```python
from build123d import *

# Parameters (mm, degrees)
BOSS_EXTRUDE1_DEPTH       = 10.287
SKETCH2_R                 = 3.556
CUT_EXTRUDE1_DEPTH        = 0.635
SKETCH3_W                 = 3.048
SKETCH3_H                 = 6.858
CUT_EXTRUDE2_DEPTH        = 0.635
SKETCH4_W                 = 6.731
SKETCH4_H                 = 1.016
CUT_EXTRUDE3_DEPTH        = 1.016
SKETCH5_W                 = 2.54
SKETCH5_H                 = 6.35
CUT_EXTRUDE4_DEPTH        = 0.635
FILLET1_R                 = 6.35
FILLET2_R                 = 2.54
CUT_EXTRUDE5_DEPTH        = 66.856694641
SKETCH9_W                 = 2.54
SKETCH9_H                 = 6.35
SKETCH9_R                 = 3.556
BOSS_EXTRUDE2_DEPTH       = 0.635
SKETCH10_W                = 6.731
SKETCH10_H                = 1.016
BOSS_EXTRUDE3_DEPTH       = 1.016
SKETCH12_W                = 3.048
SKETCH12_H                = 6.858
BOSS_EXTRUDE4_DEPTH       = 1.27
FILLET5_R                 = 0.508
FILLET5_OF_MIRROR4_R      = 0.508
F_1_0_16_DIAMETER_HOLE1_D = 4.064
SKETCH15_R                = 1.651
BOSS_EXTRUDE5_DEPTH       = 1.397
FILLET6_R                 = 1.397
SKETCH16_R                = 2.8575
BOSS_EXTRUDE6_DEPTH       = 3.302
SKETCH20_R                = 2.0701
CUT_EXTRUDE6_DEPTH        = 57.826504432
SKETCH21_W                = 8.255
SKETCH21_H                = 3.429
CUT_EXTRUDE7_DEPTH        = 3.81


with BuildPart() as part:
    # Sketch1 → Boss-Extrude1 (new, symmetric)
    with BuildSketch(Plane.XY):
        with BuildLine():
            Line((0, 0), (49.911, 0))
            Line((49.911, 0), (49.911, 23.368))
            Line((49.911, 23.368), (-5.1435, 23.368))
            ThreePointArc((-5.1435, 23.368), (-10.795, 17.7165), (-5.1435, 12.065))
            Line((-5.1435, 12.065), (0, 12.065))
            Line((0, 12.065), (0, 0))
        make_face()
    extrude(amount=BOSS_EXTRUDE1_DEPTH, both=True)

    # Sketch2 → Cut-Extrude1 (cut)
    with BuildSketch(Plane.XY.offset(10.287)):
        with Locations((-5.1435, 17.7165)):
            Circle(SKETCH2_R)
    cut_extrude1 = extrude(amount=-CUT_EXTRUDE1_DEPTH, mode=Mode.SUBTRACT)

    # Mirror1: Cut-Extrude1 across plane
    add(cut_extrude1.mirror(Plane.XY), mode=Mode.SUBTRACT)

    # Sketch3 → Cut-Extrude2 (cut)
    with BuildSketch(Plane.XY.offset(10.287)):
        with Locations((46.228, 8.89)):
            Rectangle(SKETCH3_W, SKETCH3_H)
    cut_extrude2 = extrude(amount=-CUT_EXTRUDE2_DEPTH, mode=Mode.SUBTRACT)

    # Sketch4 → Cut-Extrude3 (cut)
    with BuildSketch(Plane.XY.offset(10.287)):
        with Locations((38.7985, 20.32)):
            Rectangle(SKETCH4_W, SKETCH4_H)
    cut_extrude3 = extrude(amount=-CUT_EXTRUDE3_DEPTH, mode=Mode.SUBTRACT)

    # Sketch5 → Cut-Extrude4 (cut)
    with BuildSketch(Plane.XY.offset(10.287)):
        with Locations((24.892, 16.891)):
            Rectangle(SKETCH5_W, SKETCH5_H)
    cut_extrude4 = extrude(amount=-CUT_EXTRUDE4_DEPTH, mode=Mode.SUBTRACT)

    # Mirror2: Cut-Extrude2, Cut-Extrude3, Cut-Extrude4 across plane
    add(cut_extrude2.mirror(Plane.XY), mode=Mode.SUBTRACT)
    add(cut_extrude3.mirror(Plane.XY), mode=Mode.SUBTRACT)
    add(cut_extrude4.mirror(Plane.XY), mode=Mode.SUBTRACT)

    # Fillet1
    fillet1_edges = [part.edges().sort_by_distance(p)[0] for p in [
        (49.911, 23.368, 0),
    ]]
    fillet(fillet1_edges, radius=FILLET1_R)

    # Fillet2
    fillet2_edges = [part.edges().sort_by_distance(p)[0] for p in [
        (0, 12.065, 0),
        (24.9555, 0, -10.287),
        (24.9555, 0, 10.287),
    ]]
    fillet(fillet2_edges, radius=FILLET2_R)

    # Sketch8 → Cut-Extrude5 (cut, through all)
    with BuildSketch(Plane(origin=(49.911, 0, 0), x_dir=(0, 0, -1), z_dir=(1, 0, 0))):
        with BuildLine():
            Line((-8.763, 23.368), (-8.763, 2.54))
            ThreePointArc((-8.763, 2.54), (-8.46542049, 1.82157951), (-7.747, 1.524))
            Line((-7.747, 1.524), (7.747, 1.524))
            ThreePointArc((7.747, 1.524), (8.46542049, 1.82157951), (8.763, 2.54))
            Line((8.763, 2.54), (8.763, 23.368))
            Line((8.763, 23.368), (-8.763, 23.368))
        make_face()
    extrude(amount=-CUT_EXTRUDE5_DEPTH, mode=Mode.SUBTRACT)

    # Sketch9 → Boss-Extrude2 (add)
    with BuildSketch(Plane(origin=(0, 0, 8.763), x_dir=(-1, 0, 0), z_dir=(0, 0, -1))):
        with Locations((-24.892, 16.891)):
            Rectangle(SKETCH9_W, SKETCH9_H)
        with Locations(Location((5.1435, 17.7165, 0), (0, 0, 180))):
            Circle(SKETCH9_R)
    boss_extrude2 = extrude(amount=BOSS_EXTRUDE2_DEPTH)

    # Sketch10 → Boss-Extrude3 (add)
    with BuildSketch(Plane(origin=(0, 0, 8.763), x_dir=(-1, 0, 0), z_dir=(0, 0, -1))):
        with Locations((-38.7985, 20.32)):
            Rectangle(SKETCH10_W, SKETCH10_H)
    boss_extrude3 = extrude(amount=BOSS_EXTRUDE3_DEPTH)

    # Sketch12 → Boss-Extrude4 (add)
    with BuildSketch(Plane(origin=(0, 0, 8.763), x_dir=(-1, 0, 0), z_dir=(0, 0, -1))):
        with Locations((-46.228, 8.89)):
            Rectangle(SKETCH12_W, SKETCH12_H)
    boss_extrude4 = extrude(amount=BOSS_EXTRUDE4_DEPTH)

    # Fillet5
    fillet5_edges = [part.edges().sort_by_distance(p)[0] for p in [
        (26.162, 16.891, 8.128),
        (24.892, 13.716, 8.128),
        (23.622, 16.891, 8.128),
        (24.892, 20.066, 8.128),
        (-8.6995, 17.7165, 8.128),
        (38.7985, 20.828, 7.747),
        (42.164, 20.32, 7.747),
        (38.7985, 19.812, 7.747),
        (35.433, 20.32, 7.747),
        (46.228, 12.319, 7.493),
        (47.752, 8.89, 7.493),
        (46.228, 5.461, 7.493),
        (44.704, 8.89, 7.493),
    ]]
    fillet(fillet5_edges, radius=FILLET5_R - 0.0001)  # a hair under: the kernel refuses the full size

    # Mirror4: Boss-Extrude2, Boss-Extrude3, Boss-Extrude4 across plane
    add(boss_extrude2.mirror(Plane.XY))
    add(boss_extrude3.mirror(Plane.XY))
    add(boss_extrude4.mirror(Plane.XY))

    # Fillet5 of Mirror4
    fillet5_of_mirror4_edges = [part.edges().sort_by_distance(p)[0] for p in [
        (26.162, 16.891, -8.128),
        (24.892, 13.716, -8.128),
        (23.622, 16.891, -8.128),
        (24.892, 20.066, -8.128),
        (-8.6995, 17.7165, -8.128),
        (38.7985, 20.828, -7.747),
        (42.164, 20.32, -7.747),
        (38.7985, 19.812, -7.747),
        (35.433, 20.32, -7.747),
        (46.228, 12.319, -7.493),
        (47.752, 8.89, -7.493),
        (46.228, 5.461, -7.493),
        (44.704, 8.89, -7.493),
    ]]
    fillet(fillet5_of_mirror4_edges, radius=FILLET5_OF_MIRROR4_R - 0.0001)  # a hair under: the kernel refuses the full size

    # 1 (0.16) Diameter Hole1 (through all)
    with Locations(Plane.XY.offset(9.652)):
        with Locations((-5.1435, 17.7165)):
            Hole(F_1_0_16_DIAMETER_HOLE1_D / 2)

    # Sketch15 → Boss-Extrude5 (add)
    with BuildSketch(Plane.XZ):
        with Locations(Location((4.9911, 0, 0), (0, 0, 90))):
            Circle(SKETCH15_R)
        with Locations(Location((44.6786, 0, 0), (0, 0, 90))):
            Circle(SKETCH15_R)
    extrude(amount=BOSS_EXTRUDE5_DEPTH)

    # Fillet6
    fillet6_edges = [part.edges().sort_by_distance(p)[0] for p in [
        (4.9911, -1.397, -1.651),
        (44.6786, -1.397, -1.651),
    ]]
    fillet(fillet6_edges, radius=FILLET6_R - 0.0001)  # a hair under: the kernel refuses the full size

    # Sketch16 → Boss-Extrude6 (add)
    with BuildSketch(Plane.XZ.offset(-1.524)):
        with Locations(Location((13.0556, 0, 0), (0, 0, 90))):
            Circle(SKETCH16_R)
        with Locations(Location((36.6141, 0, 0), (0, 0, 90))):
            Circle(SKETCH16_R)
    extrude(amount=BOSS_EXTRUDE6_DEPTH)

    # Sketch20 → Cut-Extrude6 (cut, through all)
    with BuildSketch(Plane.XZ.offset(1.778)):
        with Locations(Location((13.0556, 0, 0), (0, 0, 270))):
            Circle(SKETCH20_R)
        with Locations(Location((36.6141, 0, 0), (0, 0, 270))):
            Circle(SKETCH20_R)
    extrude(amount=-CUT_EXTRUDE6_DEPTH, mode=Mode.SUBTRACT)

    # Sketch21 → Cut-Extrude7 (cut)
    with BuildSketch(Plane.XY.offset(10.287)):
        with Locations((40.0685, 1.7145)):
            Rectangle(SKETCH21_W, SKETCH21_H)
    cut_extrude7 = extrude(amount=-CUT_EXTRUDE7_DEPTH, mode=Mode.SUBTRACT)

    # Mirror5: Cut-Extrude7 across plane
    add(cut_extrude7.mirror(Plane.XY), mode=Mode.SUBTRACT)


solid = part.part
```
Model file for the job. Use its own axes, mm. A direction names the side the tool comes from. Give positions to 0.01 mm unless a question says otherwise; leave off trailing zeros. Loops run counter-clockwise (first coordinate to the right, second up) from the corner with the lowest first, then second, coordinate; pieces in that order, holes last. Notation, with made-up numbers: (-23.75, 86.25) - (33.25, 86.25) arc R32 cw to (33.25, 113.25) - close; hole circle Ø8 at (-32.75, 87.5). An arc over 180 degrees is marked (long way). One line per item, written item: value. Start each with the question number.
1. Slice it at A-A (x = 29.5). List the corners of the cut face in (y, z), plus the area to 3 significant figures.
2. Which spindle directions (+Z, -Z, +X, -X, +Y, -Y) get a long thin tool onto all of the face, cutting with end or side? Do faces 4 (the flat face through (-2.8, 17.8, 9.652)), 5 (the flat face through (40, 1, -6.477)), 6 (the flat face through (20, 13, -8.763)), 7 (the flat face through (46, 9, 7.493)), 8 (the flat face through (-5, 20, 8.128)). Say none if no direction does.
3. Probe L1, parallel to X at y = 0.35, z = 0; L2, parallel to Z at x = 46, y = 3; L3, parallel to X at y = 0.5, z = -7.5. List the from-to ranges inside material, lowest first. Write a range as from..to.
4. Pull direction Y, two halves, no side cores. Call faces 1 (the cylindrical face through (-0.724, 11.301, 9.514)), 2 (the cylindrical face through (-5.914, 14.245, 9.974)), 3 (the flat face through (46, 9, -7.493)): pulls with the +Y half, pulls with the -Y half, needs draft (parallel to the pull), parting line crosses it, or undercut.
5. Pin check, flat tips, straight feed: pin 1 (0.7 mm diameter, centred on y = 18.5, z = 10, fed in from -X); pin 2 (0.8 mm diameter, centred on y = 10.5, z = 8.5, fed in from -X); pin 3 (1.2 mm diameter, centred on x = 24.5, y = 16.5, fed in from -Z); pin 4 (3.5 mm diameter, centred on x = -5.14, y = 17.72, fed in from +Z). Stop position of each tip, or through.
6. Slice it at D-D (x = -6.5). Give the number of separate pieces and of enclosed holes in the cut face, plus the area to 3 significant figures.
7. Slice it at C-C (z = -4.5). List the corners of the cut face in (x, y).
8. Slice it at B-B (y = 10.25). List the corners of the cut face in (x, z).
Solution:
1. outline: (0, -7.75) arc R2.54 ccw to (2.54, -10.29) - (23.37, -10.29) - (23.37, -8.76) - (2.54, -8.76) arc R1.02 cw to (1.52, -7.75) - (1.52, 7.75) arc R1.02 cw to (2.54, 8.76) - (23.37, 8.76) - (23.37, 10.29) - (2.54, 10.29) arc R2.54 ccw to (0, 7.75) - close
1. area: 95.6 mm^2
2. face 4: +Z
2. face 5: -Z, +Y, -Y
2. face 6: none
2. face 7: +X, -X, +Y
2. face 8: -X, +Y, -Y
3. L1: x = 0..10.99, 15.13..34.54, 38.68..49.91
3. L2: z = -10.29..-8.76, 8.76..10.29
3. L3: x = 0..35.94, 44.2..49.91
4. face 1: pulls with the -Y half
4. face 2: undercut
4. face 3: needs draft
5. pin 1: stops at x = -10.78
5. pin 2: stops at x = -0.34
5. pin 3: stops at z = -9.65
5. pin 4: passes through
6. separate pieces: 4
6. enclosed holes: 0
6. area: 24.0 mm^2
7. outline: (0, 0) - (49.91, 0) - (49.91, 1.52) - (0, 1.52) - close
8. outline: (-0.11, -10.29) - (44.7, -10.29) - (44.7, -9.65) - (47.75, -9.65) - (47.75, -10.29) - (49.91, -10.29) - (49.91, -8.76) - (47.75, -8.76) - (47.75, -8) arc R0.51 ccw to (47.24, -7.49) - (45.21, -7.49) arc R0.51 ccw to (44.7, -8) - (44.7, -8.76) - (-0.11, -8.76) - close; (-0.11, 8.76) - (44.7, 8.76) - (44.7, 8) arc R0.51 ccw to (45.21, 7.49) - (47.24, 7.49) arc R0.51 ccw to (47.75, 8) - (47.75, 8.76) - (49.91, 8.76) - (49.91, 10.29) - (47.75, 10.29) - (47.75, 9.65) - (44.7, 9.65) - (44.7, 10.29) - (-0.11, 10.29) - close
